from build123d import *

# Parameters (mm, degrees)
SKETCH1_W                 = 101.6
SKETCH1_H                 = 101.6
BOSS_EXTRUDE1_DEPTH       = 25
SHELL1_T                  = -2
SHELL1_THICKNESS_2_FACE_W = 97.6
SHELL1_THICKNESS_2_FACE_H = 23
SHELL1_THICKNESS_2_DEPTH  = 8
SHELL1_THICKNESS_3_FACE_W = 97.6
SHELL1_THICKNESS_3_FACE_H = 23
SHELL1_THICKNESS_3_DEPTH  = 8
SKETCH2_W                 = 5
SKETCH2_H                 = 15
CUT_EXTRUDE1_DEPTH        = 25
CUT_EXTRUDE2_DEPTH        = 117.310790557
FILLET2_R                 = 3
FILLET3_R                 = 2
CUT_EXTRUDE4_DEPTH        = 77.067601513
CUT_EXTRUDE7_START        = -99.6
SKETCH11_W                = 2.3
SKETCH11_H                = 18
CUT_EXTRUDE7_DEPTH        = 17.710790557
SKETCH12_W                = 81.6
SKETCH12_H                = 2.25
CUT_EXTRUDE8_DEPTH        = 10
BOSS_EXTRUDE2_DEPTH       = 2
BOSS_EXTRUDE3_DEPTH       = 2
FILLET4_R                 = 2
FILLET4_OF_MIRROR1_R      = 2
FILLET5_R                 = 5


with BuildPart() as part:
    # Sketch1 → Boss-Extrude1 (new body)
    with BuildSketch(Plane(origin=(0, 0, 0), x_dir=(1, 0, 0), z_dir=(0, 1, 0))):
        Rectangle(SKETCH1_W, SKETCH1_H)
    extrude(amount=BOSS_EXTRUDE1_DEPTH)

    # Shell1
    shell1_openings = [part.faces().sort_by_distance(p)[0] for p in [
        (0, 25, 0),
    ]]
    offset(amount=SHELL1_T, openings=shell1_openings, kind=Kind.INTERSECTION)

    # Shell1 thickness 2 face (on inner face of the shell) → Shell1 thickness 2 (add)
    with BuildSketch(Plane(origin=(48.8, 13.5, 0), x_dir=(0, 0, 1), z_dir=(1, 0, 0))):
        Rectangle(SHELL1_THICKNESS_2_FACE_W, SHELL1_THICKNESS_2_FACE_H)
    extrude(amount=-SHELL1_THICKNESS_2_DEPTH)

    # Shell1 thickness 3 face (on inner face of the shell) → Shell1 thickness 3 (add)
    with BuildSketch(Plane(origin=(-48.8, 13.5, 0), x_dir=(0, 0, -1), z_dir=(-1, 0, 0))):
        Rectangle(SHELL1_THICKNESS_3_FACE_W, SHELL1_THICKNESS_3_FACE_H)
    extrude(amount=-SHELL1_THICKNESS_3_DEPTH)

    # Sketch2 → Cut-Extrude1 (cut)
    with BuildSketch(Plane(origin=(0, 2, 0), x_dir=(1, 0, 0), z_dir=(0, 1, 0))):
        with Locations((0, 37.3)):
            Rectangle(SKETCH2_W, SKETCH2_H)
    extrude(amount=-CUT_EXTRUDE1_DEPTH, mode=Mode.SUBTRACT)

    # Sketch3 → Cut-Extrude2 (cut, through all)
    with BuildSketch(Plane(origin=(50.8, 0, 0), x_dir=(0, 0, -1), z_dir=(1, 0, 0))):
        with BuildLine():
            Line((-15, 42), (15, 42))
            Line((15, 42), (15, 10))
            ThreePointArc((15, 10), (14.414213562, 8.585786438), (13, 8))
            Line((13, 8), (-13, 8))
            ThreePointArc((-13, 8), (-14.414213562, 8.585786438), (-15, 10))
            Line((-15, 10), (-15, 42))
        make_face()
    extrude(amount=-CUT_EXTRUDE2_DEPTH, mode=Mode.SUBTRACT)

    # Fillet2
    fillet2_edges = [part.edges().sort_by_distance(p)[0] for p in [
        (-40.8, 13.5, -48.8),
        (-40.8, 13.5, 48.8),
        (40.8, 13.5, 48.8),
        (40.8, 13.5, -48.8),
    ]]
    fillet(fillet2_edges, radius=FILLET2_R)

    # Fillet3
    fillet3_edges = [part.edges().sort_by_distance(p)[0] for p in [
        (40.8, 2, 0),
        (-40.8, 2, 0),
        (0, 2, 48.8),
        (0, 2, -48.8),
        (-39.921320344, 2, -47.921320344),
        (-39.921320344, 2, 47.921320344),
        (39.921320344, 2, 47.921320344),
        (39.921320344, 2, -47.921320344),
    ]]
    fillet(fillet3_edges, radius=FILLET3_R)

    # Sketch7 → Cut-Extrude4 (cut, through all)
    with BuildSketch(Plane(origin=(0, 25, 0), x_dir=(1, 0, 0), z_dir=(0, 1, 0))):
        Polygon((51, -31), (48.882842712, -31), (45.8, -34.082842712), (42.6, -30.882842712), (42.6, -20.717157288), (45.8, -17.517157288), (48.882842712, -20.6), (51, -20.6), align=None)
        Polygon((-51, -20.6), (-51, -31), (-48.882842712, -31), (-45.8, -34.082842712), (-42.6, -30.882842712), (-42.6, -20.717157288), (-45.8, -17.517157288), (-48.882842712, -20.6), align=None)
        Polygon((-51, 31), (-48.882842712, 31), (-45.8, 34.082842712), (-42.6, 30.882842712), (-42.6, 20.717157288), (-45.8, 17.517157288), (-48.882842712, 20.6), (-51, 20.6), align=None)
        Polygon((51, 20.6), (51, 31), (48.882842712, 31), (45.8, 34.082842712), (42.6, 30.882842712), (42.6, 20.717157288), (45.8, 17.517157288), (48.882842712, 20.6), align=None)
    extrude(amount=-CUT_EXTRUDE4_DEPTH, mode=Mode.SUBTRACT)

    # Sketch11 → Cut-Extrude7 (cut, through all)
    with BuildSketch(Plane(origin=(0, 0, -50.8), x_dir=(-1, 0, 0), z_dir=(0, 0, -1)).offset(CUT_EXTRUDE7_START)):
        with Locations((-20.8, 16)):
            Rectangle(SKETCH11_W, SKETCH11_H)
        with Locations((20.8, 16)):
            Rectangle(SKETCH11_W, SKETCH11_H)
        with BuildLine():
            Line((-13, 4), (13, 4))
            ThreePointArc((13, 4), (14.414213562, 4.585786438), (15, 6))
            Line((15, 6), (15, 18))
            ThreePointArc((15, 18), (14.414213562, 19.414213562), (13, 20))
            Line((13, 20), (-13, 20))
            ThreePointArc((-13, 20), (-14.414213562, 19.414213562), (-15, 18))
            Line((-15, 18), (-15, 6))
            ThreePointArc((-15, 6), (-14.414213562, 4.585786438), (-13, 4))
        make_face()
    extrude(amount=-CUT_EXTRUDE7_DEPTH, mode=Mode.SUBTRACT)

    # Sketch12 → Cut-Extrude8 (cut)
    with BuildSketch(Plane(origin=(0, 0, -50.8), x_dir=(-1, 0, 0), z_dir=(0, 0, -1))):
        with Locations((0, 23.875)):
            Rectangle(SKETCH12_W, SKETCH12_H)
    extrude(amount=-CUT_EXTRUDE8_DEPTH, mode=Mode.SUBTRACT)

    # Sketch13 → Boss-Extrude2 (add)
    with BuildSketch(Plane(origin=(0, 22.75, 0), x_dir=(1, 0, 0), z_dir=(0, 1, 0))):
        with BuildLine():
            Line((40.8, 45.8), (40.8, 15))
            Line((40.8, 15), (37.8, 15))
            Line((37.8, 15), (37.8, 48.8))
            ThreePointArc((37.8, 48.8), (39.921320344, 47.921320344), (40.8, 45.8))
        make_face()
        with BuildLine():
            Line((40.8, -45.8), (40.8, -15))
            Line((40.8, -15), (37.8, -15))
            Line((37.8, -15), (37.8, -48.8))
            ThreePointArc((37.8, -48.8), (39.921320344, -47.921320344), (40.8, -45.8))
        make_face()
    boss_extrude2 = extrude(amount=-BOSS_EXTRUDE2_DEPTH)

    # Sketch14 → Boss-Extrude3 (add)
    with BuildSketch(Plane(origin=(0, 25, 0), x_dir=(1, 0, 0), z_dir=(0, 1, 0))):
        Polygon((50.8, 50.8), (35.8, 50.8), (35.8, 15), (50.8, 15), (50.8, 20.6), (48.882842712, 20.6), (45.8, 17.517157288), (42.6, 20.717157288), (42.6, 30.882842712), (45.8, 34.082842712), (48.882842712, 31), (50.8, 31), align=None)
        Polygon((21.95, -50.8), (21.95, -48.8), (35.8, -48.8), (35.8, -15), (50.8, -15), (50.8, -20.6), (48.882842712, -20.6), (45.8, -17.517157288), (42.6, -20.717157288), (42.6, -30.882842712), (45.8, -34.082842712), (48.882842712, -31), (50.8, -31), (50.8, -50.8), align=None)
    boss_extrude3 = extrude(amount=BOSS_EXTRUDE3_DEPTH)

    # Fillet4
    fillet4_edges = [part.edges().sort_by_distance(p)[0] for p in [
        (35.8, 26, 48.8),
    ]]
    fillet(fillet4_edges, radius=FILLET4_R)

    # Mirror1: Boss-Extrude2, Boss-Extrude3 across plane
    add(boss_extrude2.mirror(Plane(origin=(0, 0, 0), x_dir=(0, 0, 1), z_dir=(1, 0, 0))))
    add(boss_extrude3.mirror(Plane(origin=(0, 0, 0), x_dir=(0, 0, 1), z_dir=(1, 0, 0))))

    # Fillet4 of Mirror1
    fillet4_of_mirror1_edges = [part.edges().sort_by_distance(p)[0] for p in [
        (-35.8, 26, 48.8),
    ]]
    fillet(fillet4_of_mirror1_edges, radius=FILLET4_OF_MIRROR1_R)

    # Fillet5
    fillet5_edges = [part.edges().sort_by_distance(p)[0] for p in [
        (0, 0, -50.8),
    ]]
    fillet(fillet5_edges, radius=FILLET5_R)


solid = part.part
Can you work these out from the model? Positions are in its coordinate system, mm. A direction names the side the tool comes from. Give positions to 0.01 mm unless a question says otherwise; leave off trailing zeros. Order: outer loops, then holes, each group sorted by start corner. A loop starts at its lowest first (then second) coordinate and runs counter-clockwise, first axis right, second up. Notation, with made-up numbers: M 34.5,78.25 L 92.5,78.25 A14 ccw 92.5,86.25 Z; hole C -2,0.25 d8. An arc over 180 degrees is marked long. Use a Markdown table: item, result. Add a question column.
Item 1: We'd pull the mould along Z, two halves only. Please class faces 4 (the flat face through (-50.8, 13, 41)), 5 (the flat face through (45, 18, -15)), 6 (the flat face through (-1, 13, -50.8)), 7 (the flat face through (-42.6, 14, 26)): +Z half, -Z half, draft (parallel to the pull), parting line (faces both ways), or undercut.
Item 2: Suppose I cut it at A-A (x = -5). List the corners of the cut face in (y, z) for me.
Item 3: Suppose I cut it at B-B (z = -28.5). List the corners of the cut face in (x, y) for me, then the cut area to 3 significant figures.
Item 4: If I drill on L1, parallel to Z at x = 33, y = 7.5; L2, parallel to X at y = 16.5, z = -29; L3, parallel to Z at x = 41.5, y = 16, over which ranges is the centre line in solid material (lowest first)? Write a range as [from, to].
Item 5: For faces 1 (the flat face through (-42.6, 13, -26)), 2 (the flat face through (-38, 25, -33)), 3 (the flat face through (39, 20.75, 32)), which set-ups out of +Z, -Z, +X, -X, +Y, -Y let a thin tool reach every point of the face, with its end or its side?
Item 6: Will these pins go through, and if not, where does the flat tip stop? pin 1 (1 mm diameter, centred on x = -1, y = 1.5, fed in from -Z); pin 2 (12 mm diameter, centred on x = -19.5, z = 16.5, fed in from +Y); pin 3 (1 mm diameter, centred on y = 22, z = 29, fed in from +X).
Item 7: Suppose I cut it at D-D (x = 27). List the corners of the cut face in (y, z) for me, then the cut area to 3 significant figures.
Item 8: Suppose I cut it at C-C (y = 14.25). Count the separate pieces of the cut face and the enclosed holes in it, then the cut area to 3 significant figures.
Answer sheet:
| question | item | result |
|---|---|---|
| 1 | face 4 | draft |
| 1 | face 5 | undercut |
| 1 | face 6 | -Z half |
| 1 | face 7 | undercut |
| 2 | outline | M 0,-45.8 A5 ccw 5,-50.8 L 22.75,-50.8 L 22.75,-48.8 L 4,-48.8 A2 cw 2,-46.8 L 2,46.8 A2 cw 4,48.8 L 4,50.8 L 0,50.8 Z; M 20,48.8 L 25,48.8 L 25,50.8 L 20,50.8 Z |
| 3 | outline | M -42.6,0 L 42.6,0 L 42.6,27 L 35.8,27 L 35.8,25 L 40.8,25 L 40.8,22.75 L 37.8,22.75 L 37.8,20.75 L 40.8,20.75 L 40.8,4 A2 cw 38.8,2 L -38.8,2 A2 cw -40.8,4 L -40.8,20.75 L -37.8,20.75 L -37.8,22.75 L -40.8,22.75 L -40.8,25 L -35.8,25 L -35.8,27 L -42.6,27 Z |
| 3 | area | 294 mm² |
| 4 | L1 | z = [-50.8, -48.8], [48.8, 50.8] |
| 4 | L2 | x = [-42.6, -40.8], [40.8, 42.6] |
| 4 | L3 | z = [-50.8, -15], [15, 50.8] |
| 5 | face 1 | -X, +Y, -Y |
| 5 | face 2 | -Z |
| 5 | face 3 | none |
| 6 | pin 1 | stops at z = -49.8 |
| 6 | pin 2 | stops at y = 2 |
| 6 | pin 3 | stops at x = 42.6 |
| 7 | outline | M 0,-45.8 A5 ccw 5,-50.8 L 22.75,-50.8 L 22.75,-48.8 L 4,-48.8 A2 cw 2,-46.8 L 2,46.8 A2 cw 4,48.8 L 27,48.8 L 27,50.8 L 0,50.8 Z |
| 7 | area | 291 mm² |
| 8 | separate pieces | 5 |
| 8 | enclosed holes | 0 |
| 8 | area | 1,280 mm² |
